```python
from build123d import *

# Parameters (mm, degrees)
BOSS_EXTRUDE1_DEPTH                                  = 5.08
FILLET1_R                                            = 6.35
SKETCH2_R                                            = 2.00025
CUT_EXTRUDE1_DEPTH                                   = 5.08
CUT_EXTRUDE2_DEPTH                                   = 1.524
CSK_FOR_M3_HEX_SOCKET_COUNTERSUNK_CAP_SC_D           = 3.4
CSK_FOR_M3_HEX_SOCKET_COUNTERSUNK_CAP_SC_CSINK_D     = 6.72
CSK_FOR_M3_HEX_SOCKET_COUNTERSUNK_CAP_SC_CSINK_ANGLE = 90


with BuildPart() as part:
    # Sketch1 → Boss-Extrude1 (new body)
    with BuildSketch(Plane.XY):
        with BuildLine():
            Line((-38.1, -44.45), (38.1, -44.45))
            ThreePointArc((38.1, -44.45), (42.590128061, -42.590128061), (44.45, -38.1))
            Line((44.45, -38.1), (44.45, 38.1))
            ThreePointArc((44.45, 38.1), (42.590128061, 42.590128061), (38.1, 44.45))
            Line((38.1, 44.45), (-38.1, 44.45))
            ThreePointArc((-38.1, 44.45), (-42.590128061, 42.590128061), (-44.45, 38.1))
            Line((-44.45, 38.1), (-44.45, -38.1))
            ThreePointArc((-44.45, -38.1), (-42.590128061, -42.590128061), (-38.1, -44.45))
        make_face()
    extrude(amount=BOSS_EXTRUDE1_DEPTH)

    # Fillet1
    # the kernel refuses this fillet: 6.35 mm, written as the material it takes off along each edge
    with BuildSketch(Plane(origin=(38.1, 44.45, 5.08), x_dir=(0, -1.563753501140824e-12, -1.0), z_dir=(-1, 0, 0)), Plane(origin=(44.45, -38.1, 5.08), x_dir=(-1.563753501140824e-12, 0, -1.0), z_dir=(0, 1, 0)), Plane(origin=(-38.1, -44.45, 5.08), x_dir=(0, 1.563753501140824e-12, -1.0), z_dir=(1, 0, 0)), Plane(origin=(-44.45, 38.1, 5.08), x_dir=(1.563753501140824e-12, 0, -1.0), z_dir=(0, -1, 0))) as fillet1_piece_1:
        with BuildLine():
            CenterArc((6.35, 6.221703947), FILLET1_R, 180, 78.463040967)
            Line((0, 6.221703947), (-0.127, 6.221703947))
            Line((-0.127, 6.221703947), (-0.127, 0))
            Line((-0.127, 0), (0, -0.127))
            ThreePointArc((0, -0.127), (2.54, -0.127), (5.0546, -0.124434079))
            Line((5.0546, -0.124434079), (5.08, 0))
        make_face()
    extrude(amount=76.2, mode=Mode.SUBTRACT)
    with BuildSketch(Plane(origin=(38.1, 38.1, 5.08), x_dir=(1, 0, 0), z_dir=(0, -1, 0))) as fillet1_piece_2:
        with BuildLine():
            CenterArc((0.128296053, -6.35), FILLET1_R, 11.536959033, 78.463040967)
            Line((0.128296053, 0), (0.128296053, 0.127))
            Line((0.128296053, 0.127), (6.35, 0.127))
            Line((6.35, 0.127), (6.477, 0))
            ThreePointArc((6.477, 0), (6.477, -2.54), (6.474434079, -5.0546))
            Line((6.474434079, -5.0546), (6.35, -5.08))
        make_face()
    revolve(axis=Axis((38.1, 38.1, 5.08), (0, 0, 1)), revolution_arc=90, mode=Mode.SUBTRACT)
    with BuildSketch(Plane(origin=(38.1, -38.1, 5.08), x_dir=(0, -1, 0), z_dir=(-1, 0, 0))) as fillet1_piece_3:
        with BuildLine():
            CenterArc((0.128296053, -6.35), FILLET1_R, 11.536959033, 78.463040967)
            Line((0.128296053, 0), (0.128296053, 0.127))
            Line((0.128296053, 0.127), (6.35, 0.127))
            Line((6.35, 0.127), (6.477, 0))
            ThreePointArc((6.477, 0), (6.477, -2.54), (6.474434079, -5.0546))
            Line((6.474434079, -5.0546), (6.35, -5.08))
        make_face()
    revolve(axis=Axis((38.1, -38.1, 5.08), (0, 0, 1)), revolution_arc=90, mode=Mode.SUBTRACT)
    with BuildSketch(Plane(origin=(-38.1, -38.1, 5.08), x_dir=(-1, 0, 0), z_dir=(0, 1, 0))) as fillet1_piece_4:
        with BuildLine():
            CenterArc((0.128296053, -6.35), FILLET1_R, 11.536959033, 78.463040967)
            Line((0.128296053, 0), (0.128296053, 0.127))
            Line((0.128296053, 0.127), (6.35, 0.127))
            Line((6.35, 0.127), (6.477, 0))
            ThreePointArc((6.477, 0), (6.477, -2.54), (6.474434079, -5.0546))
            Line((6.474434079, -5.0546), (6.35, -5.08))
        make_face()
    revolve(axis=Axis((-38.1, -38.1, 5.08), (0, 0, 1)), revolution_arc=90, mode=Mode.SUBTRACT)
    with BuildSketch(Plane(origin=(-38.1, 38.1, 5.08), x_dir=(0, 1, 0), z_dir=(1, 0, 0))) as fillet1_piece_5:
        with BuildLine():
            CenterArc((0.128296053, -6.35), FILLET1_R, 11.536959033, 78.463040967)
            Line((0.128296053, 0), (0.128296053, 0.127))
            Line((0.128296053, 0.127), (6.35, 0.127))
            Line((6.35, 0.127), (6.477, 0))
            ThreePointArc((6.477, 0), (6.477, -2.54), (6.474434079, -5.0546))
            Line((6.474434079, -5.0546), (6.35, -5.08))
        make_face()
    revolve(axis=Axis((-38.1, 38.1, 5.08), (0, 0, 1)), revolution_arc=90, mode=Mode.SUBTRACT)

    # Sketch2 → Cut-Extrude1 (cut)
    with BuildSketch(Plane.XY.offset(5.08)):
        with Locations(Location((-36.83, 36.83, 0), (0, 0, 44.351687845))):
            Circle(SKETCH2_R)
        with Locations(Location((36.83, 36.83, 0), (0, 0, 39.414098339))):
            Circle(SKETCH2_R)
        with Locations(Location((36.83, -36.83, 0), (0, 0, 320.585901644))):
            Circle(SKETCH2_R)
        with Locations(Location((-36.83, -36.83, 0), (0, 0, 315.648312155))):
            Circle(SKETCH2_R)
    extrude(amount=-CUT_EXTRUDE1_DEPTH, mode=Mode.SUBTRACT)

    # Sketch4 → Cut-Extrude2 (cut)
    with BuildSketch(Plane(origin=(0, 0, 0), x_dir=(-1, 0, 0), z_dir=(0, 0, -1))):
        Polygon((-9.779, 9.779), (-9.779, 34.925), (9.779, 34.925), (9.779, 9.779), (34.925, 9.779), (34.925, -9.779), (9.779, -9.779), (9.779, -34.925), (-9.779, -34.925), (-9.779, -9.779), (-34.925, -9.779), (-34.925, 9.779), align=None)
    extrude(amount=-CUT_EXTRUDE2_DEPTH, mode=Mode.SUBTRACT)

    # CSK for M3 Hex Socket Countersunk Cap Screw1 (through all)
    with Locations(Plane.XY.offset(5.08)):
        with Locations((-36.83, 36.83), (36.83, 36.83), (36.83, -36.83), (-36.83, -36.83)):
            CounterSinkHole(CSK_FOR_M3_HEX_SOCKET_COUNTERSUNK_CAP_SC_D / 2, CSK_FOR_M3_HEX_SOCKET_COUNTERSUNK_CAP_SC_CSINK_D / 2, counter_sink_angle=CSK_FOR_M3_HEX_SOCKET_COUNTERSUNK_CAP_SC_CSINK_ANGLE)


solid = part.part
```
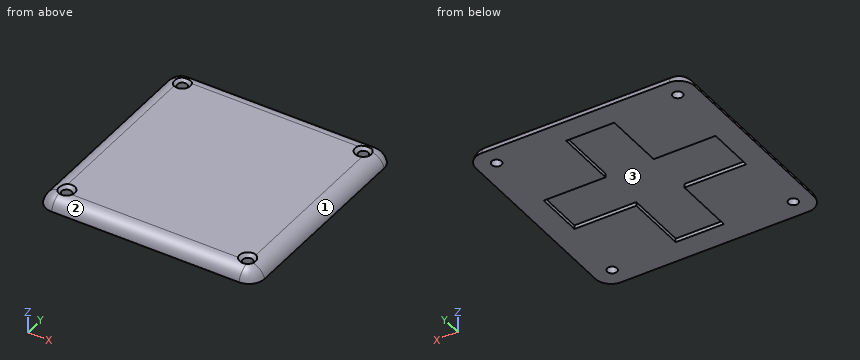
CAD build for the part. Positions are in the model's coordinates, mm. Face numbers are marked on the shaded views. Coordinates: 2 decimals unless noted, no trailing zeros. Write each loop counter-clockwise with the first axis right and the second up, starting at its lowest first coordinate (ties: lowest second). Pieces come first, ordered by that corner, then holes.
(1) Two-plate mould, pull along X, no slides. Class the marked faces 1, 2 and 3: +X half, -X half, draft (parallel to the pull), parting line (faces both ways), or undercut.
(2) Cut at D-D, the plane x = -25.5. List the corners of the cut face in (y, z), and give its area (3 significant figures).
(3) Cut at A-A, the plane x = 36.83. List the corners of the cut face in (y, z).
(4) Drill centre lines: probe 1 along Y at (x, z) = (-36.83, 1); probe 2 along Y at (x, z) = (-36.83, 2.85); probe 3 along X at (y, z) = (36.83, 0.8). Where is each one in solid material? Low to high.
(5) Flat gauge pins, fed straight in: pin 1 (0.8 mm diameter, centred on y = -1.5, z = 0.5, fed in from -X); pin 2 (4.5 mm diameter, centred on x = 36.83, y = 36.83, fed in from +Z); pin 3 (2 mm diameter, centred on y = 28.5, z = 1.5, fed in from +X); pin 4 (3.5 mm diameter, centred on x = -36.83, y = 36.83, fed in from -Z). Where does each tip first touch, or does it go through?
(6) Cut at B-B, the plane y = 7. List the corners of the cut face in (x, z) (3 decimals), and give its area (3 significant figures).
Geometry says:
1. face 1: +X half
1. face 2: draft
1. face 3: undercut
2. outline: (-44.45, 0) - (-9.78, 0) - (-9.78, 1.52) - (9.78, 1.52) - (9.78, 0) - (44.45, 0) arc R6.35 ccw to (38.23, 5.08) - (-38.23, 5.08) arc R6.35 ccw to start
2. area: 406 mm2
3. outline: (-44.45, 0) - (-38.83, 0) - (-38.83, 3.72) - (-39.95, 4.84) arc R6.35 ccw to start; (-34.83, 0) - (34.83, 0) - (34.83, 3.72) - (33.47, 5.08) - (-33.47, 5.08) - (-34.83, 3.72) - close; (38.83, 0) - (44.45, 0) arc R6.35 ccw to (39.95, 4.84) - (38.83, 3.72) - close
4. probe 1: y = -44.16 to -38.83, -34.83 to 34.83, 38.83 to 44.16
4. probe 2: y = -43.06 to -38.83, -34.83 to 34.83, 38.83 to 43.06
4. probe 3: x = -44.23 to -38.83, -34.83 to 34.83, 38.83 to 44.23
5. pin 1: stops at x = -44.43
5. pin 2: stops at z = 3.97
5. pin 3: stops at x = 44.33
5. pin 4: passes through
6. outline: (-44.45, 0) - (-34.925, 0) - (-34.925, 1.524) - (34.925, 1.524) - (34.925, 0) - (44.45, 0) arc R6.35 ccw to (38.228, 5.08) - (-38.228, 5.08) arc R6.35 ccw to start
6. area: 329 mm2
